Autodesk Inventor part; units mm, degrees
ref_plane "YZ Plane" through (0, 0, 0) normal (1, 0, 0) x (0, 1, 0)
ref_plane "XZ Plane" through (0, 0, 0) normal (0, 1, 0) x (-1, 0, 0)
ref_plane "XY Plane" through (0, 0, 0) normal (0, 0, 1) x (1, 0, 0)
sketch "Sketch1" plane through (0, 0, 0) normal (0, 1, 0) x (-1, 0, 0)
  arc A0 (-30.0072, 97.3212) -> (-35.8309, 103.5589) centre (-41.895, 92.0599) ccw
  arc A1 (-30.286, 94.3964) -> (-30.0072, 97.3212) centre (-32.7505, 96.107) ccw
  arc A2 (-30.286, 94.3964) -> (-31, 92.1156) centre (-27, 92.1156) ccw
  line L0 (-31, 92.1156) -> (-31, 77.1156)
  arc A3 (-31, 77.1156) -> (-30.286, 74.8348) centre (-27, 77.1156) ccw
  arc A4 (-30.0072, 71.9101) -> (-30.286, 74.8348) centre (-32.7505, 73.1242) ccw
  arc A5 (-35.8309, 65.6723) -> (-30.0072, 71.9101) centre (-41.895, 77.1713) ccw
  arc A6 (-35.8309, 65.6723) -> (-34.9925, 43.1559) centre (-30, 54.6156) ccw
  arc A7 (-27.7949, 35.1735) -> (-34.9925, 43.1559) centre (-40.1848, 31.2379) ccw
  line L1 (-27.7949, 35.1735) -> (-17.0958, 1.4913)
  arc A8 (-17.0958, 1.4913) -> (-14.6505, -1.0569) centre (-13.2835, 2.7022) ccw
  line L2 (-14.6505, -1.0569) -> (-2.0505, -5.6388)
  arc A9 (-2.0505, -5.6388) -> (2.0505, -5.6388) centre (0, 0) ccw
  line L3 (2.0505, -5.6388) -> (14.6505, -1.0569)
  arc A10 (14.6505, -1.0569) -> (17.0958, 1.4913) centre (13.2835, 2.7022) ccw
  line L4 (17.0958, 1.4913) -> (27.7949, 35.1735)
  arc A11 (34.9925, 43.1559) -> (27.7949, 35.1735) centre (40.1848, 31.2379) ccw
  arc A12 (34.9925, 43.1559) -> (35.8309, 65.6723) centre (30, 54.6156) ccw
  arc A13 (30.0072, 71.9101) -> (35.8309, 65.6723) centre (41.895, 77.1713) ccw
  arc A14 (30.286, 74.8348) -> (30.0072, 71.9101) centre (32.7505, 73.1242) ccw
  arc A15 (30.286, 74.8348) -> (31, 77.1156) centre (27, 77.1156) ccw
  line L5 (31, 77.1156) -> (31, 92.1156)
  arc A16 (31, 92.1156) -> (30.286, 94.3964) centre (27, 92.1156) ccw
  arc A17 (30.0072, 97.3212) -> (30.286, 94.3964) centre (32.7505, 96.107) ccw
  arc A18 (35.8309, 103.5589) -> (30.0072, 97.3212) centre (41.895, 92.0599) ccw
  arc A19 (35.8309, 103.5589) -> (21.1612, 123.4545) centre (30, 114.6156) ccw
  line L6 (21.1612, 123.4545) -> (13.9152, 116.2085)
  arc A20 (13.9152, 116.2085) -> (11.0366, 112.9476) centre (38.6639, 91.4597) ccw
  line L7 (11.0366, 112.9476) -> (3.1574, 102.8173)
  arc A21 (-3.1574, 102.8173) -> (3.1574, 102.8173) centre (0, 105.273) ccw
  line L8 (-3.1574, 102.8173) -> (-11.0366, 112.9476)
  arc A22 (-11.0366, 112.9476) -> (-13.9152, 116.2085) centre (-38.6639, 91.4597) ccw
  line L9 (-13.9152, 116.2085) -> (-21.1612, 123.4545)
  arc A23 (-21.1612, 123.4545) -> (-35.8309, 103.5589) centre (-30, 114.6156) ccw
  arc A24 (25.5, 77.1156) -> (28.5, 77.1156) centre (27, 77.1156) ccw
  line L10 (25.5, 92.1156) -> (25.5, 77.1156)
  arc A25 (28.5, 92.1156) -> (25.5, 92.1156) centre (27, 92.1156) ccw
  line L11 (28.5, 77.1156) -> (28.5, 92.1156)
  arc A26 (-28.5, 77.1156) -> (-25.5, 77.1156) centre (-27, 77.1156) ccw
  line L12 (-28.5, 92.1156) -> (-28.5, 77.1156)
  arc A27 (-25.5, 92.1156) -> (-28.5, 92.1156) centre (-27, 92.1156) ccw
  line L13 (-25.5, 77.1156) -> (-25.5, 92.1156)
  circle A28 centre (-30, 54.6156) radius 1.5
  circle A29 centre (-13.2835, 2.7022) radius 1.5
  circle A30 centre (-25.4558, 101.5862) radius 1.5
  circle A31 centre (-25.4558, 67.6451) radius 1.5
  circle A32 centre (-15, 99.6156) radius 3
  circle A33 centre (25.4558, 67.6451) radius 1.5
  circle A34 centre (25.4558, 101.5862) radius 1.5
  circle A35 centre (15, 69.6156) radius 3
  circle A36 centre (30, 54.6156) radius 1.5
  circle A37 centre (30, 114.6156) radius 1.5
  circle A38 centre (24.2029, 37.0782) radius 1.5
  circle A39 centre (13.2835, 2.7022) radius 1.5
  circle A40 centre (16.9706, 110.0715) radius 1.5
  circle A41 centre (16.9706, 59.1598) radius 1.5
  circle A42 centre (15, 99.6156) radius 3
  circle A43 centre (-15, 69.6156) radius 3
  circle A44 centre (-16.9706, 59.1598) radius 1.5
  circle A45 centre (-16.9706, 110.0715) radius 1.5
  circle A46 centre (-24.2029, 37.0782) radius 1.5
  circle A47 centre (-30, 114.6156) radius 1.5
  point P0 (-30.286, 94.3964)
  point P1 (-35.8309, 65.6723)
  point P2 (-34.9925, 43.1559)
  point P3 (-27.7949, 35.1735)
  point P4 (-17.0958, 1.4913)
  point P5 (-14.6505, -1.0569)
  point P6 (2.0505, -5.6388)
  point P7 (14.6505, -1.0569)
  point P8 (27.7949, 35.1735)
  point P9 (35.8309, 65.6723)
  point P10 (30.0072, 71.9101)
  point P11 (30.286, 74.8348)
  point P12 (30.286, 94.3964)
  point P13 (30.0072, 97.3212)
  point P14 (13.9152, 116.2085)
  point P15 (11.0366, 112.9476)
  point P16 (-3.1574, 102.8173)
  point P17 (-13.9152, 116.2085)
  point P18 (-21.1612, 123.4545)
  point P19 (-35.8309, 103.5589)
  point P20 (-30.0072, 97.3212)
  point P21 (25.5, 77.1156)
  point P22 (28.5, 77.1156)
extrude "Extrusion1" add sketch "Sketch1" along normal blind 3
sketch "Sketch2" plane through (0, 3, 0) normal (0, 1, 0) x (1, 0, 0)
  line L0 (31, -92.1156) -> (31, -77.1156) construction
  arc A0 (31, -77.1156) -> (30.286, -74.8348) centre (27, -77.1156) ccw construction
  arc A1 (30.0072, -71.9101) -> (30.286, -74.8348) centre (32.7505, -73.1242) ccw construction
  arc A2 (35.8309, -65.6723) -> (30.0072, -71.9101) centre (41.895, -77.1713) ccw construction
  arc A3 (35.8309, -65.6723) -> (34.9925, -43.1559) centre (30, -54.6156) ccw construction
  arc A4 (27.7949, -35.1735) -> (34.9925, -43.1559) centre (40.1848, -31.2379) ccw construction
  line L1 (27.7949, -35.1735) -> (17.0958, -1.4913) construction
  arc A5 (17.0958, -1.4913) -> (14.6505, 1.0569) centre (13.2835, -2.7022) ccw construction
  line L2 (14.6505, 1.0569) -> (2.0505, 5.6388) construction
  arc A6 (2.0505, 5.6388) -> (-2.0505, 5.6388) centre (0, 0) ccw construction
  line L3 (-2.0505, 5.6388) -> (-14.6505, 1.0569) construction
  arc A7 (-14.6505, 1.0569) -> (-17.0958, -1.4913) centre (-13.2835, -2.7022) ccw construction
  line L4 (-17.0958, -1.4913) -> (-27.7949, -35.1735) construction
  arc A8 (-34.9925, -43.1559) -> (-27.7949, -35.1735) centre (-40.1848, -31.2379) ccw construction
  arc A9 (-34.9925, -43.1559) -> (-35.8309, -65.6723) centre (-30, -54.6156) ccw construction
  arc A10 (-30.0072, -71.9101) -> (-35.8309, -65.6723) centre (-41.895, -77.1713) ccw construction
  arc A11 (-30.286, -74.8348) -> (-30.0072, -71.9101) centre (-32.7505, -73.1242) ccw construction
  arc A12 (-30.286, -74.8348) -> (-31, -77.1156) centre (-27, -77.1156) ccw construction
  line L5 (-31, -77.1156) -> (-31, -92.1156) construction
  arc A13 (-31, -92.1156) -> (-30.286, -94.3964) centre (-27, -92.1156) ccw construction
  arc A14 (-30.0072, -97.3212) -> (-30.286, -94.3964) centre (-32.7505, -96.107) ccw construction
  arc A15 (-35.8309, -103.5589) -> (-30.0072, -97.3212) centre (-41.895, -92.0599) ccw construction
  arc A16 (-35.8309, -103.5589) -> (-21.1612, -123.4545) centre (-30, -114.6156) ccw construction
  line L6 (-21.1612, -123.4545) -> (-13.9152, -116.2085) construction
  arc A17 (-13.9152, -116.2085) -> (-11.0366, -112.9476) centre (-38.6639, -91.4597) ccw construction
  line L7 (-11.0366, -112.9476) -> (-3.1574, -102.8173) construction
  arc A18 (3.1574, -102.8173) -> (-3.1574, -102.8173) centre (0, -105.273) ccw construction
  line L8 (3.1574, -102.8173) -> (11.0366, -112.9476) construction
  arc A19 (11.0366, -112.9476) -> (13.9152, -116.2085) centre (38.6639, -91.4597) ccw construction
  line L9 (13.9152, -116.2085) -> (21.1612, -123.4545) construction
  arc A20 (21.1612, -123.4545) -> (35.8309, -103.5589) centre (30, -114.6156) ccw construction
  arc A21 (30.0072, -97.3212) -> (35.8309, -103.5589) centre (41.895, -92.0599) ccw construction
  arc A22 (30.286, -94.3964) -> (30.0072, -97.3212) centre (32.7505, -96.107) ccw construction
  arc A23 (30.286, -94.3964) -> (31, -92.1156) centre (27, -92.1156) ccw construction
  circle A24 centre (25.4558, -101.5862) radius 1.5 construction
  circle A25 centre (-16.9706, -110.0715) radius 1.5
  circle A26 centre (-15, -99.6156) radius 3 construction
  circle A27 centre (-15, -69.6156) radius 3 construction
  circle A28 centre (-24.2029, -37.0782) radius 1.5 construction
  circle A29 centre (24.2029, -37.0782) radius 1.5 construction
  circle A30 centre (15, -69.6156) radius 3 construction
  circle A31 centre (16.9706, -59.1598) radius 1.5 construction
  circle A32 centre (30, -54.6156) radius 1.5 construction
  circle A33 centre (25.4558, -67.6451) radius 1.5 construction
  circle A34 centre (16.9706, -110.0715) radius 1.5
  circle A35 centre (15, -99.6156) radius 3 construction
  circle A36 centre (-25.4558, -67.6451) radius 1.5 construction
  circle A37 centre (-16.9706, -59.1598) radius 1.5 construction
  circle A38 centre (-25.4558, -101.5862) radius 1.5 construction
  circle A39 centre (-30, -54.6156) radius 1.5 construction
  circle A40 centre (-13.2835, -2.7022) radius 1.5 construction
  circle A41 centre (13.2835, -2.7022) radius 1.5 construction
  circle A42 centre (30, -114.6156) radius 1.5
  line L10 (-25.5, -77.1156) -> (-25.5, -92.1156) construction
  arc A43 (-28.5, -92.1156) -> (-25.5, -92.1156) centre (-27, -92.1156) ccw construction
  line L11 (-28.5, -92.1156) -> (-28.5, -77.1156) construction
  arc A44 (-25.5, -77.1156) -> (-28.5, -77.1156) centre (-27, -77.1156) ccw construction
  circle A45 centre (-30, -114.6156) radius 1.5
  line L12 (28.5, -77.1156) -> (28.5, -92.1156) construction
  arc A46 (25.5, -92.1156) -> (28.5, -92.1156) centre (27, -92.1156) ccw construction
  line L13 (25.5, -92.1156) -> (25.5, -77.1156) construction
  arc A47 (28.5, -77.1156) -> (25.5, -77.1156) centre (27, -77.1156) ccw construction
  circle A48 centre (16.9706, -110.0715) radius 5 construction
  circle A49 centre (-16.9706, -110.0715) radius 5 construction
  arc A50 (-31.1155, -107.199) -> (-30, -122.1156) centre (-30, -114.6156) ccw
  arc A51 (30, -122.1156) -> (31.1155, -107.199) centre (30, -114.6156) ccw
  line L14 (30, -122.1156) -> (-30, -122.1156)
  line L15 (-16.9706, -105.0715) -> (16.9706, -105.0715)
  line L16 (-16.9706, -105.0715) -> (-31.1155, -107.199)
  line L17 (16.9706, -105.0715) -> (31.1155, -107.199)
  arc A52 (31.1155, -107.199) -> (30, -122.1156) centre (30, -114.6156) ccw construction
  arc A53 (-30, -122.1156) -> (-31.1155, -107.199) centre (-30, -114.6156) ccw construction
  line L18 (0, -105.273) -> (0, -113.6943) construction
  line L19 (0, -113.6943) -> (3.1574, -113.6943) construction
  line L20 (0, -113.6943) -> (0, -122.1156) construction
  circle A54 centre (0, -109.4837) radius 1.55
  line L21 (0, -117.905) -> (15.6117, -117.905) construction
  line L22 (13.9152, -116.2085) -> (21.1612, -123.4545)
  line L23 (0, -117.905) -> (-15.6117, -117.905) construction
  line L24 (-21.1612, -123.4545) -> (-13.9152, -116.2085)
  circle A55 centre (7.8058, -117.905) radius 1.55
  circle A56 centre (-7.8058, -117.905) radius 1.55
  dimension "d2" = 10
  dimension "d3" = 10
  dimension "d4" = 15
  dimension "d5" = 15
  dimension "d8" = 3.1
  dimension "d9" = 3.1
  dimension "d10" = 3.1
extrude "Extrusion2" [suppressed]
properties part number "399 prig z plate"
Model file for the job. Use its own axes, mm. A direction names the side the tool comes from. Round coordinates to 2 decimals unless told otherwise and drop trailing zeros. Write each loop counter-clockwise with the first axis right and the second up, starting at its lowest first coordinate (ties: lowest second). Pieces come first, ordered by that corner, then holes. Notation, with made-up numbers: (-34.5, 23) - (-16.5, 23) arc R32 ccw to (-16.5, 62) - close; hole circle Ø11 at (24.25, -20.75). An arc over 180 degrees is marked (long way). Use CSV: the item, a comma, the result in double quotes. Start each with the question number.
Item 1: Pin check, flat tips, straight feed: P1, Ø2, axis at x = 0, z = 51, coming from the -Y side; P2, Ø0.9, axis at y = 1.5, z = 84.5, coming from the +X side; P3, Ø1, axis at x = -7, y = 1, coming from the -Z side. Stop position of each tip, or through.
Item 2: Tool access for faces 4 (the face through (12.45, 1.48, 114.65)), 5 (the face through (-31, 1, 85)), 6 (the face through (-27.033, 1.479, 75.616)), 7 (the face through (0, 1, -6)): list every direction of +Z, -Z, +X, -X, +Y, -Y with a clear straight run to the whole face (end or side of a thin tool).
Item 3: Band-saw the part on A-A (y = 2.3). State how many separate pieces and enclosed holes the cut face has, and give its area (3 significant figures).
Item 4: Band-saw the part on C-C (x = -5). Write the cut outline in (y, z), and give its area (3 significant figures).
Item 5: Drill centre lines: L1, parallel to Z at x = 30, y = 2.05; L2, parallel to X at y = 1.8, z = 69; L3, parallel to Z at x = 29.5, y = 2.85. Where is each one in solid material? Low to high. Write a range as [from, to].
Item 6: Two-plate mould, pull along Z, no slides. Class faces 1 (the face through (22.52, 1.48, 18.57)), 2 (the face through (16.16, 1.48, 108.81)), 3 (the face through (17.487, 1.479, 119.781)): released by +Z, released by -Z, zero draft, split by the parting line, or undercut.
Item 7: Band-saw the part on B-B (z = 5.5). Write the cut outline in (x, y).
Checked values:
1,P1,"stops at y = 0"
1,P2,"stops at x = 31"
1,P3,"stops at z = -4.02"
2,face 4,"+Z, +Y, -Y"
2,face 5,"-X, +Y, -Y"
2,face 6,"+Y, -Y"
2,face 7,"-Z, +Y, -Y"
3,separate pieces,"1"
3,enclosed holes,"22"
3,area,"7,250 mm²"
4,outline,"(0, -4.57) - (3, -4.57) - (3, 105.19) - (0, 105.19) - close"
4,area,"329 mm²"
5,L1,"z = [39.32, 53.12], [56.12, 71.93], [74.32, 94.91], [97.3, 113.12], [116.12, 127.12]"
5,L2,"x = [-31.78, -26.1], [-24.81, -17.94], [-12.06, 12.06], [17.94, 24.81], [26.1, 31.78]"
5,L3,"z = [38.64, 53.2], [56.03, 113.2], [116.03, 127.11]"
6,face 1,"released by -Z"
6,face 2,"undercut"
6,face 3,"released by +Z"
7,outline,"(-18.37, 0) - (18.37, 0) - (18.37, 3) - (-18.37, 3) - close"
